Could you check a few things on this model? Use its own coordinates, in mm. A direction names the side the tool comes from. Give positions to 0.01 mm unless a question says otherwise; leave off trailing zeros. Return JSON: item names as keys, results as strings. Group by question number.
1. If we mould it in two halves opening along Y, with no side actions, what happens to faces 3 (the flat face through (-1, -64, 0)), 4 (the flat face through (9, -115, 2)), 5 (the cylindrical face through (-10.01, 15.57, 2.48)), 6 (the flat face through (-1, -150.2, 2))? For each: +Y half, -Y half, draft (parallel to the pull), parting line (faces both ways), or undercut.
2. If we section it at A-A (z = 2.45): State how many separate pieces and enclosed holes the cut face has, plus the area to 3 significant figures.
3. Please list where these lines run through material, in increasing order: line 1 (X direction, y = -144.2, z = 2.3); line 2 (Y direction, x = -1, z = 2.7); line 3 (X direction, y = -12, z = 2.35).
4. For faces 1 (the flat face through (19.9, -76, 2)), 2 (the flat face through (6.3, 1, 2)), which set-ups out of +Z, -Z, +X, -X, +Y, -Y let a thin tool reach every point of the face, with its end or its side?
5. For pin 1 (1.2 mm diameter, centred on y = 1, z = 3, fed in from -X); pin 2 (4.5 mm diameter, centred on x = -8.75, y = -12.43, fed in from -Z); pin 3 (4 mm diameter, centred on x = -8.75, y = 14.43, fed in from -Z), each with a flat end and sliding along its axis, tell me the tip position at first contact or that it passes through.
```python
from build123d import *

# Parameters (mm, degrees)
SKETCH1_W           = 41.8
SKETCH1_H           = 170
SKETCH1_R           = 1.7
SKETCH1_R_2         = 3.5
BOSS_EXTRUDE1_DEPTH = 4
FILLET1_R           = 20
SKETCH2_R           = 1.7
DEPENDANT_DEPTH     = 10
CHAMFER1_SIZE       = 1


with BuildPart() as part:
    # Sketch1 → Boss-Extrude1 (new body)
    with BuildSketch(Plane.XY):
        with Locations((-1, -65.2)):
            Rectangle(SKETCH1_W, SKETCH1_H)
        with Locations((6.748548523, -12.425907791)):
            Circle(SKETCH1_R, mode=Mode.SUBTRACT)
        with Locations((-8.754354431, -12.425907791)):
            Circle(SKETCH1_R, mode=Mode.SUBTRACT)
        with Locations((-16.505805908, 1)):
            Circle(SKETCH1_R, mode=Mode.SUBTRACT)
        with Locations((-8.754354431, 14.425907791)):
            Circle(SKETCH1_R, mode=Mode.SUBTRACT)
        with Locations((6.748548523, 14.425907791)):
            Circle(SKETCH1_R, mode=Mode.SUBTRACT)
        with Locations((14.5, 1)):
            Circle(SKETCH1_R, mode=Mode.SUBTRACT)
        with Locations((14, -144.2)):
            Circle(SKETCH1_R, mode=Mode.SUBTRACT)
        with Locations((-16, -144.2)):
            Circle(SKETCH1_R, mode=Mode.SUBTRACT)
        with Locations((-1, -133.2)):
            Circle(SKETCH1_R_2, mode=Mode.SUBTRACT)
        with BuildLine():
            Line((6.3, 8), (6.3, -6))
            ThreePointArc((6.3, -6), (-1, -13.3), (-8.3, -6))
            Line((-8.3, -6), (-8.3, 8))
            ThreePointArc((-8.3, 8), (-1, 15.3), (6.3, 8))
        make_face(mode=Mode.SUBTRACT)
        with BuildLine():
            Line((-9, -121.2), (7, -121.2))
            ThreePointArc((7, -121.2), (8.414213562, -120.614213562), (9, -119.2))
            Line((9, -119.2), (9, -111.2))
            ThreePointArc((9, -111.2), (8.414213562, -109.785786438), (7, -109.2))
            Line((7, -109.2), (-9, -109.2))
            ThreePointArc((-9, -109.2), (-10.414213562, -109.785786438), (-11, -111.2))
            Line((-11, -111.2), (-11, -119.2))
            ThreePointArc((-11, -119.2), (-10.414213562, -120.614213562), (-9, -121.2))
        make_face(mode=Mode.SUBTRACT)
    extrude(amount=BOSS_EXTRUDE1_DEPTH)

    # Fillet1
    fillet1_edges = [part.edges().sort_by_distance(p)[0] for p in [
        (-21.9, 19.8, 2),
        (19.9, 19.8, 2),
    ]]
    fillet(fillet1_edges, radius=FILLET1_R)

    # Sketch2 → dependant (cut)
    with BuildSketch(Plane.XY.offset(4)):
        with Locations((-1, -79.702564777)):
            Circle(SKETCH2_R)
        with Locations((5.062177826, -69.202564777)):
            Circle(SKETCH2_R)
        with Locations((-7.062177826, -69.202564777)):
            Circle(SKETCH2_R)
    extrude(amount=-DEPENDANT_DEPTH, mode=Mode.SUBTRACT)

    # Chamfer1
    chamfer1_edges = [part.edges().sort_by_distance(p)[0] for p in [
        (5.048548523, -12.425907791, 0),
        (-10.454354431, -12.425907791, 0),
        (-18.205805908, 1, 0),
        (-10.454354431, 14.425907791, 0),
        (5.048548523, 14.425907791, 0),
        (12.8, 1, 0),
        (12.3, -144.2, 0),
        (-17.7, -144.2, 0),
    ]]
    chamfer(chamfer1_edges, length=CHAMFER1_SIZE)


solid = part.part
```
Answer:
{
 "1": {"face 3": "draft", "face 4": "undercut", "face 5": "undercut", "face 6": "-Y half"},
 "2": {"separate pieces": "1", "enclosed holes": "14", "area": "6,190 mm²"},
 "3": {"line 1": "x = -21.9 to -17.7, -14.3 to 12.3, 15.7 to 19.9", "line 2": "y = -150.2 to -136.7, -129.7 to -121.2, -109.2 to -81.4, -78 to -13.3, 15.3 to 19.8", "line 3": "x = -21.9 to -10.4, -7.11 to -5.16, 3.16 to 5.1, 8.39 to 19.9"},
 "4": {"face 1": "+Z, -Z, +X, +Y, -Y", "face 2": "+Z, -Z"},
 "5": {"pin 1": "stops at x = -21.89", "pin 2": "stops at z = 0.44", "pin 3": "stops at z = 0.69"}
}
